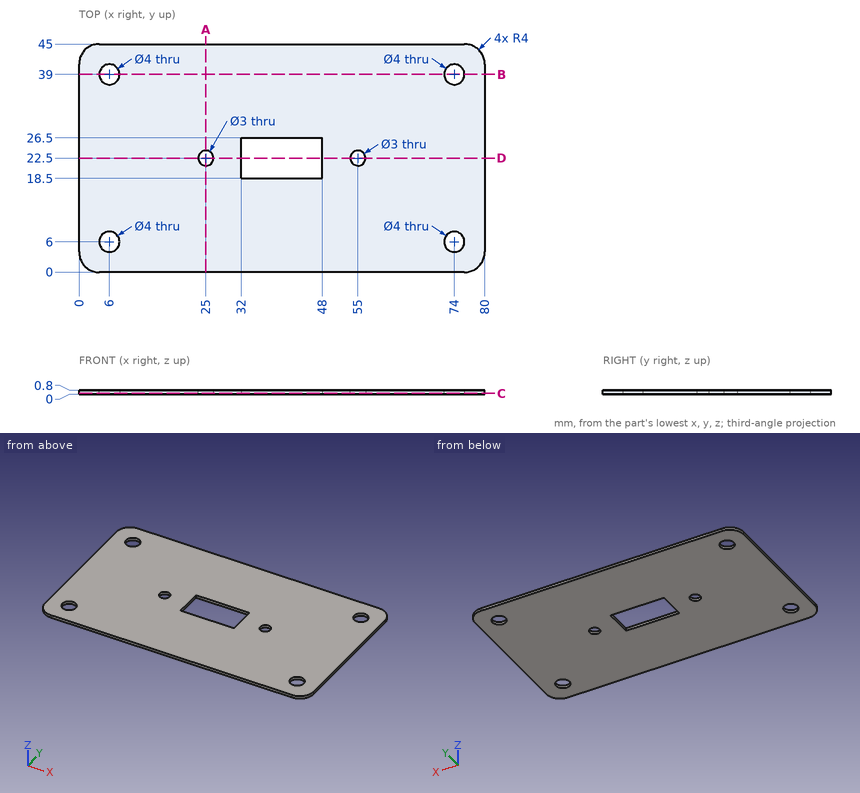
For this review, use the dimensioned drawing (mm, ordinates from the lowest corner) and the shaded views. Give positions to 0.01 mm unless a question says otherwise; leave off trailing zeros. Order: outer loops, then holes, each group sorted by start corner. A loop starts at its lowest first (then second) coordinate and runs counter-clockwise, first axis right, second up. Notation, with made-up numbers: (76.25, 88) - (92.25, 88) arc R17 cw to (92.25, 113) - close; hole circle Ø8 at (69, 20.5). An arc over 180 degrees is marked (long way). Write item = value, one per line. Start each with the question number.
Q1. We need section C-C on z = 0.2. State the section outline as (x, y) points, plus the area to 3 significant figures.
Q2. We need section A-A on x = 25. State the section outline as (y, z) points.
Q3. To check wall thickness, follow L1, parallel to Y at x = 6, z = 0.6; L2, parallel to Y at x = 46.5, z = 0.7; L3, parallel to Y at x = 55, z = 0.45. State the ranges of each line that lie inside material, in increasing order. Write a range as from..to.
Q4. We need section D-D on y = 22.5. State the section outline as (x, z) points, plus the area to 3 significant figures.
Q5. We need section B-B on y = 39. State the section outline as (x, z) points.
Working result:
q1.outline = (0, 4) arc R4 ccw to (4, 0) - (76, 0) arc R4 ccw to (80, 4) - (80, 41) arc R4 ccw to (76, 45) - (4, 45) arc R4 ccw to (0, 41) - close; hole circle Ø4 at (6, 6); hole circle Ø4 at (6, 39); hole circle Ø3 at (25, 22.5); hole (32, 18.5) - (48, 18.5) - (48, 26.5) - (32, 26.5) - close; hole circle Ø3 at (55, 22.5); hole circle Ø4 at (74, 6); hole circle Ø4 at (74, 39)
q1.area = 3,390 mm²
q2.outline = (0, 0) - (21, 0) - (21, 0.8) - (0, 0.8) - close; (24, 0) - (45, 0) - (45, 0.8) - (24, 0.8) - close
q3.L1 = 0..4, 8..37, 41..45
q3.L2 = 0..18.5, 26.5..45
q3.L3 = 0..21, 24..45
q4.outline = (0, 0) - (23.5, 0) - (23.5, 0.8) - (0, 0.8) - close; (26.5, 0) - (32, 0) - (32, 0.8) - (26.5, 0.8) - close; (48, 0) - (53.5, 0) - (53.5, 0.8) - (48, 0.8) - close; (56.5, 0) - (80, 0) - (80, 0.8) - (56.5, 0.8) - close
q4.area = 46.4 mm²
q5.outline = (0, 0) - (4, 0) - (4, 0.8) - (0, 0.8) - close; (8, 0) - (72, 0) - (72, 0.8) - (8, 0.8) - close; (76, 0) - (80, 0) - (80, 0.8) - (76, 0.8) - close
